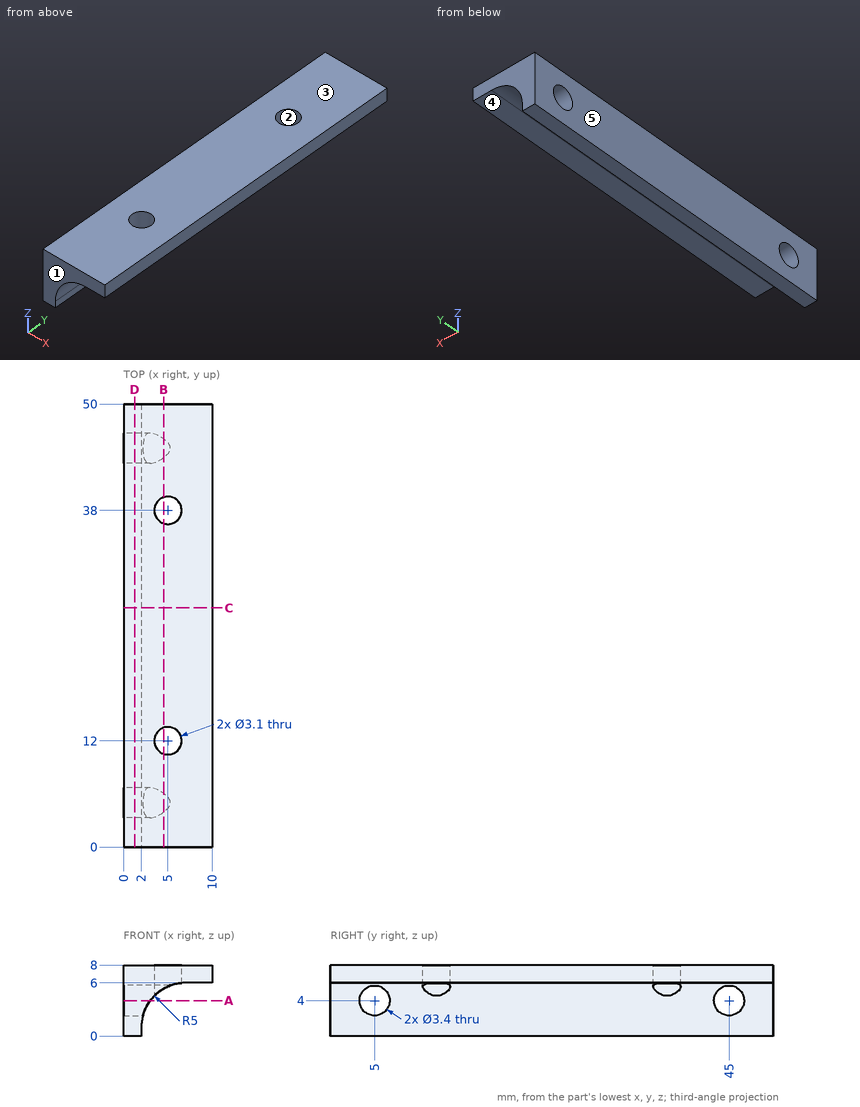
Here's the drawing with two shaded views (mm, measured from the low corner). I have some questions. A direction names the side the tool comes from. Coordinates: 2 decimals unless noted, no trailing zeros. Loops run counter-clockwise (first coordinate to the right, second up) from the corner with the lowest first, then second, coordinate; pieces in that order, holes last. Notation, with made-up numbers: M 86,-8.5 L 103,-8.5 A27 ccw 103,30.5 Z; hole C 52.25,-10 d1. An arc over 180 degrees is marked long. Put each result on its own line as item: value. Start each with the question number.
(1) Imagine slicing it at B-B on x = 4.5. List the corners of the cut face in (y, z) for me, and give its area (3 significant figures).
(2) Imagine slicing it at D-D on x = 1.25. List the corners of the cut face in (y, z) for me.
(3) Which directions (+Z, -Z, +X, -X, +Y, -Y) give clear straight access to the entire face, cutting with the end or side of a thin tool? Please do the marked faces 4 and 5.
(4) Imagine slicing it at A-A on z = 4. List the corners of the cut face in (x, y) for me, and give its area (3 significant figures).
(5) I need wall thicknesses on probe 1 along Y at (x, z) = (1.65, 4); probe 2 along Y at (x, z) = (5, 6.7); probe 3 along X at (y, z) = (34, 0.5). Which ranges of each line are inside material? Lowest first, please.
(6) We'd pull the mould along Y, two halves only. Please class the marked faces 1, 2 and 3: +Y half, -Y half, draft (parallel to the pull), parting line (faces both ways), or undercut.
(7) Will these pins go through, and if not, where does the flat tip stop? pin 1 Ø1 at (x, y) = (8.5, 39.5) entering from -Z; pin 2 Ø0.8 at (y, z) = (36, 0.5) entering from +X.
(8) Imagine slicing it at C-C on y = 27. List the corners of the cut face in (x, z) for me.
Worked answers:
1. outline: M 0,5.33 L 3.94,5.33 A1.7 cw 6.06,5.33 L 10.53,5.33 L 10.53,8 L 0,8 Z; M 13.47,5.33 L 36.53,5.33 L 36.53,8 L 13.47,8 Z; M 39.47,5.33 L 43.94,5.33 A1.7 cw 46.06,5.33 L 50,5.33 L 50,8 L 39.47,8 Z
1. area: 117 mm2
2. outline: M 0,0 L 50,0 L 50,8 L 0,8 Z; hole C 5,4 d3.4; hole C 45,4 d3.4
3. face 4: -Z, +X, +Y, -Y
3. face 5: +Z, -Z, -X, +Y, -Y
4. outline: M 0,0 L 3,0 L 3,3.3 L 0,3.3 Z; M 0,6.7 L 3,6.7 L 3,43.3 L 0,43.3 Z; M 0,46.7 L 3,46.7 L 3,50 L 0,50 Z
4. area: 130 mm2
5. probe 1: y = 0 to 3.3, 6.7 to 43.3, 46.7 to 50
5. probe 2: y = 0 to 10.45, 13.55 to 36.45, 39.55 to 50
5. probe 3: x = 0 to 2
6. face 1: -Y half
6. face 2: undercut
6. face 3: draft
7. pin 1: stops at z = 6
7. pin 2: stops at x = 2
8. outline: M 0,0 L 2,0 L 2,1 A5 cw 7,6 L 10,6 L 10,8 L 0,8 Z
